from build123d import *

# Parameters (mm, degrees)
MODEL_R                 = 1.5
SALIENTE_EXTRUIR1_DEPTH = 3


with BuildPart() as part:
    # Model → Saliente-Extruir1 (new body)
    with BuildSketch(Plane.XY):
        with BuildLine():
            Line((-1388.226934946, 304.407679238), (-1478.226934946, 304.407679238))
            ThreePointArc((-1478.226934946, 304.407679238), (-1481.408915461, 303.089659753), (-1482.726934946, 299.907679238))
            Line((-1482.726934946, 299.907679238), (-1482.726934946, 254.907679238))
            ThreePointArc((-1482.726934946, 254.907679238), (-1481.408915461, 251.725698722), (-1478.226934946, 250.407679238))
            Line((-1478.226934946, 250.407679238), (-1469.226934946, 250.407679238))
            ThreePointArc((-1469.226934946, 250.407679238), (-1466.04495443, 251.725698722), (-1464.726934946, 254.907679238))
            Line((-1464.726934946, 254.907679238), (-1464.726934946, 259.053577271))
            ThreePointArc((-1464.726934946, 259.053577271), (-1464.68680843, 259.398206652), (-1464.568575732, 259.724397665))
            Line((-1464.568575732, 259.724397665), (-1460.641524749, 267.578499631))
            ThreePointArc((-1460.641524749, 267.578499631), (-1460.088480631, 268.18365545), (-1459.299883963, 268.407679238))
            Line((-1459.299883963, 268.407679238), (-1407.153985929, 268.407679238))
            ThreePointArc((-1407.153985929, 268.407679238), (-1406.365389261, 268.18365545), (-1405.812345142, 267.578499631))
            Line((-1405.812345142, 267.578499631), (-1401.885294159, 259.724397665))
            ThreePointArc((-1401.885294159, 259.724397665), (-1401.767061462, 259.398206652), (-1401.726934946, 259.053577271))
            Line((-1401.726934946, 259.053577271), (-1401.726934946, 254.907679238))
            ThreePointArc((-1401.726934946, 254.907679238), (-1400.408915461, 251.725698722), (-1397.226934946, 250.407679238))
            Line((-1397.226934946, 250.407679238), (-1388.226934946, 250.407679238))
            ThreePointArc((-1388.226934946, 250.407679238), (-1385.04495443, 251.725698722), (-1383.726934946, 254.907679238))
            Line((-1383.726934946, 254.907679238), (-1383.726934946, 299.907679238))
            ThreePointArc((-1383.726934946, 299.907679238), (-1385.04495443, 303.089659753), (-1388.226934946, 304.407679238))
        make_face()
        with Locations((-1424.226934946, 299.907679238)):
            Circle(MODEL_R, mode=Mode.SUBTRACT)
        with Locations((-1433.226934946, 299.907679238)):
            Circle(MODEL_R, mode=Mode.SUBTRACT)
        with Locations((-1442.226934946, 299.907679238)):
            Circle(MODEL_R, mode=Mode.SUBTRACT)
        with Locations((-1478.226934946, 299.907679238)):
            Circle(MODEL_R, mode=Mode.SUBTRACT)
        with Locations((-1388.226934946, 299.907679238)):
            Circle(MODEL_R, mode=Mode.SUBTRACT)
        with Locations((-1406.226934946, 272.907679238)):
            Circle(MODEL_R, mode=Mode.SUBTRACT)
        with Locations((-1415.226934946, 272.907679238)):
            Circle(MODEL_R, mode=Mode.SUBTRACT)
        with Locations((-1424.226934946, 272.907679238)):
            Circle(MODEL_R, mode=Mode.SUBTRACT)
        with Locations((-1433.226934946, 272.907679238)):
            Circle(MODEL_R, mode=Mode.SUBTRACT)
        with Locations((-1442.226934946, 272.907679238)):
            Circle(MODEL_R, mode=Mode.SUBTRACT)
        with Locations((-1451.226934946, 272.907679238)):
            Circle(MODEL_R, mode=Mode.SUBTRACT)
        with Locations((-1460.226934946, 272.907679238)):
            Circle(MODEL_R, mode=Mode.SUBTRACT)
        with BuildLine():
            Line((-1458.726934946, 281.907679238), (-1458.726934946, 290.907679238))
            ThreePointArc((-1458.726934946, 290.907679238), (-1460.226934946, 292.407679238), (-1461.726934946, 290.907679238))
            Line((-1461.726934946, 290.907679238), (-1461.726934946, 281.907679238))
            ThreePointArc((-1461.726934946, 281.907679238), (-1460.226934946, 280.407679238), (-1458.726934946, 281.907679238))
        make_face(mode=Mode.SUBTRACT)
        with BuildLine():
            Line((-1449.726934946, 281.907679238), (-1449.726934946, 290.907679238))
            ThreePointArc((-1449.726934946, 290.907679238), (-1451.226934946, 292.407679238), (-1452.726934946, 290.907679238))
            Line((-1452.726934946, 290.907679238), (-1452.726934946, 281.907679238))
            ThreePointArc((-1452.726934946, 281.907679238), (-1451.226934946, 280.407679238), (-1449.726934946, 281.907679238))
        make_face(mode=Mode.SUBTRACT)
        with BuildLine():
            Line((-1440.726934946, 281.907679238), (-1440.726934946, 290.907679238))
            ThreePointArc((-1440.726934946, 290.907679238), (-1442.226934946, 292.407679238), (-1443.726934946, 290.907679238))
            Line((-1443.726934946, 290.907679238), (-1443.726934946, 281.907679238))
            ThreePointArc((-1443.726934946, 281.907679238), (-1442.226934946, 280.407679238), (-1440.726934946, 281.907679238))
        make_face(mode=Mode.SUBTRACT)
        with BuildLine():
            Line((-1431.726934946, 281.907679238), (-1431.726934946, 290.907679238))
            ThreePointArc((-1431.726934946, 290.907679238), (-1433.226934946, 292.407679238), (-1434.726934946, 290.907679238))
            Line((-1434.726934946, 290.907679238), (-1434.726934946, 281.907679238))
            ThreePointArc((-1434.726934946, 281.907679238), (-1433.226934946, 280.407679238), (-1431.726934946, 281.907679238))
        make_face(mode=Mode.SUBTRACT)
        with BuildLine():
            Line((-1422.726934946, 281.907679238), (-1422.726934946, 290.907679238))
            ThreePointArc((-1422.726934946, 290.907679238), (-1424.226934946, 292.407679238), (-1425.726934946, 290.907679238))
            Line((-1425.726934946, 290.907679238), (-1425.726934946, 281.907679238))
            ThreePointArc((-1425.726934946, 281.907679238), (-1424.226934946, 280.407679238), (-1422.726934946, 281.907679238))
        make_face(mode=Mode.SUBTRACT)
        with BuildLine():
            Line((-1413.726934946, 281.907679238), (-1413.726934946, 290.907679238))
            ThreePointArc((-1413.726934946, 290.907679238), (-1415.226934946, 292.407679238), (-1416.726934946, 290.907679238))
            Line((-1416.726934946, 290.907679238), (-1416.726934946, 281.907679238))
            ThreePointArc((-1416.726934946, 281.907679238), (-1415.226934946, 280.407679238), (-1413.726934946, 281.907679238))
        make_face(mode=Mode.SUBTRACT)
        with BuildLine():
            Line((-1404.726934946, 281.907679238), (-1404.726934946, 290.907679238))
            ThreePointArc((-1404.726934946, 290.907679238), (-1406.226934946, 292.407679238), (-1407.726934946, 290.907679238))
            Line((-1407.726934946, 290.907679238), (-1407.726934946, 281.907679238))
            ThreePointArc((-1407.726934946, 281.907679238), (-1406.226934946, 280.407679238), (-1404.726934946, 281.907679238))
        make_face(mode=Mode.SUBTRACT)
        with BuildLine():
            Line((-1478.226934946, 292.407679238), (-1469.226934946, 292.407679238))
            ThreePointArc((-1469.226934946, 292.407679238), (-1467.726934946, 290.907679238), (-1469.226934946, 289.407679238))
            Line((-1469.226934946, 289.407679238), (-1478.226934946, 289.407679238))
            ThreePointArc((-1478.226934946, 289.407679238), (-1479.726934946, 290.907679238), (-1478.226934946, 292.407679238))
        make_face(mode=Mode.SUBTRACT)
        with BuildLine():
            Line((-1397.226934946, 292.407679238), (-1388.226934946, 292.407679238))
            ThreePointArc((-1388.226934946, 292.407679238), (-1386.726934946, 290.907679238), (-1388.226934946, 289.407679238))
            Line((-1388.226934946, 289.407679238), (-1397.226934946, 289.407679238))
            ThreePointArc((-1397.226934946, 289.407679238), (-1398.726934946, 290.907679238), (-1397.226934946, 292.407679238))
        make_face(mode=Mode.SUBTRACT)
        with BuildLine():
            Line((-1397.226934946, 280.407679238), (-1388.226934946, 280.407679238))
            ThreePointArc((-1388.226934946, 280.407679238), (-1386.726934946, 281.907679238), (-1388.226934946, 283.407679238))
            Line((-1388.226934946, 283.407679238), (-1397.226934946, 283.407679238))
            ThreePointArc((-1397.226934946, 283.407679238), (-1398.726934946, 281.907679238), (-1397.226934946, 280.407679238))
        make_face(mode=Mode.SUBTRACT)
        with BuildLine():
            Line((-1469.226934946, 298.407679238), (-1451.226934946, 298.407679238))
            ThreePointArc((-1451.226934946, 298.407679238), (-1449.726934946, 299.907679238), (-1451.226934946, 301.407679238))
            Line((-1451.226934946, 301.407679238), (-1469.226934946, 301.407679238))
            ThreePointArc((-1469.226934946, 301.407679238), (-1470.726934946, 299.907679238), (-1469.226934946, 298.407679238))
        make_face(mode=Mode.SUBTRACT)
        with BuildLine():
            Line((-1415.226934946, 301.407679238), (-1397.226934946, 301.407679238))
            ThreePointArc((-1397.226934946, 301.407679238), (-1395.726934946, 299.907679238), (-1397.226934946, 298.407679238))
            Line((-1397.226934946, 298.407679238), (-1415.226934946, 298.407679238))
            ThreePointArc((-1415.226934946, 298.407679238), (-1416.726934946, 299.907679238), (-1415.226934946, 301.407679238))
        make_face(mode=Mode.SUBTRACT)
        with BuildLine():
            Line((-1478.226934946, 280.407679238), (-1469.226934946, 280.407679238))
            ThreePointArc((-1469.226934946, 280.407679238), (-1467.726934946, 281.907679238), (-1469.226934946, 283.407679238))
            Line((-1469.226934946, 283.407679238), (-1478.226934946, 283.407679238))
            ThreePointArc((-1478.226934946, 283.407679238), (-1479.726934946, 281.907679238), (-1478.226934946, 280.407679238))
        make_face(mode=Mode.SUBTRACT)
        with BuildLine():
            Line((-1478.226934946, 256.407679238), (-1469.226934946, 256.407679238))
            ThreePointArc((-1469.226934946, 256.407679238), (-1467.726934946, 254.907679238), (-1469.226934946, 253.407679238))
            Line((-1469.226934946, 253.407679238), (-1478.226934946, 253.407679238))
            ThreePointArc((-1478.226934946, 253.407679238), (-1479.726934946, 254.907679238), (-1478.226934946, 256.407679238))
        make_face(mode=Mode.SUBTRACT)
        with BuildLine():
            Line((-1397.226934946, 256.407679238), (-1388.226934946, 256.407679238))
            ThreePointArc((-1388.226934946, 256.407679238), (-1386.726934946, 254.907679238), (-1388.226934946, 253.407679238))
            Line((-1388.226934946, 253.407679238), (-1397.226934946, 253.407679238))
            ThreePointArc((-1397.226934946, 253.407679238), (-1398.726934946, 254.907679238), (-1397.226934946, 256.407679238))
        make_face(mode=Mode.SUBTRACT)
    extrude(amount=SALIENTE_EXTRUIR1_DEPTH)


solid = part.part
Read the model definition and answer for the solid it produces. Units are mm, in the model's axes. Coordinates: 2 decimals unless noted, no trailing zeros. Loops run counter-clockwise (first coordinate to the right, second up) from the corner with the lowest first, then second, coordinate; pieces in that order, holes last. Notation, with made-up numbers: (42, 6) - (68, 6) arc R29 ccw to (68, 37) - close; hole circle Ø8 at (-25.75, 39). An arc over 180 degrees is marked (long way). Answer in a Markdown table with one row per item.
Q1. The mould has two halves that part along Y. Classify faces 1 (the cylindrical face through (-1467.727, 281.875, 1.479)), 2 (the flat face through (-1474, 289.408, 1)), 3 (the cylindrical face through (-1385.08, 251.69, 1.48)): pulls with the +Y half, pulls with the -Y half, needs draft (parallel to the pull), parting line crosses it, or undercut.
Here are the results:
| item | result |
|---|---|
| face 1 | undercut |
| face 2 | undercut |
| face 3 | pulls with the -Y half |
Q2. Find section B-B on x = -1455.5. Write down the section's boundary in (y, z).
Here are the results:
| item | result |
|---|---|
| outline | (268.41, 0) - (298.41, 0) - (298.41, 3) - (268.41, 3) - close; (301.41, 0) - (304.41, 0) - (304.41, 3) - (301.41, 3) - close |
Q3. Find section A-A on y = 288.5. Count the separate pieces of the cut face and the enclosed holes in it, plus the area to 3 significant figures.
Here are the results:
| item | result |
|---|---|
| separate pieces | 8 |
| enclosed holes | 0 |
| area | 234 mm^2 |
Q4. Find section C-C on x = -1442. Write down the section's boundary in (y, z), plus the area to 3 significant figures.
Here are the results:
| item | result |
|---|---|
| outline | (268.41, 0) - (271.42, 0) - (271.42, 3) - (268.41, 3) - close; (274.39, 0) - (280.42, 0) - (280.42, 3) - (274.39, 3) - close; (292.39, 0) - (298.42, 0) - (298.42, 3) - (292.39, 3) - close; (301.39, 0) - (304.41, 0) - (304.41, 3) - (301.39, 3) - close |
| area | 54.3 mm^2 |
Q5. Given P1, Ø2.5, axis at x = -1424.23, y = 299.91, coming from the +Z side; P2, Ø1.5, axis at x = -1421, z = 1, coming from the -Y side, each flat-ended and moving along its own axis, determine where each tip first touches the part or whether it passes through.
Here are the results:
| item | result |
|---|---|
| P1 | passes through |
| P2 | stops at y = 268.41 |
Q6. Straight lines are drawn through the part: line 1 along Y through (x, z) = (-1388, 2.9); line 2 along Y through (x, z) = (-1454, 1.7); line 3 along Y through (x, z) = (-1415.5, 1.85). For each, find the intervals that lie inside material, in ascending order. Write a range as [from, to].
Here are the results:
| item | result |
|---|---|
| line 1 | y = [250.41, 253.42], [256.39, 280.42], [283.39, 289.42], [292.39, 298.42], [301.39, 304.4] |
| line 2 | y = [268.41, 298.41], [301.41, 304.41] |
| line 3 | y = [268.41, 271.43], [274.38, 280.43], [292.38, 298.43], [301.38, 304.41] |
